Geometry check sheet. Reference: the model listing, model coordinates, mm. Face numbers are marked on the shaded views. A direction names the side the tool comes from. Give positions to 0.01 mm unless a question says otherwise; leave off trailing zeros. Write each loop counter-clockwise with the first axis right and the second up, starting at its lowest first coordinate (ties: lowest second). Pieces come first, ordered by that corner, then holes. Notation, with made-up numbers: (29, 13) - (72, 13) arc R32 ccw to (72, 48) - close; hole circle Ø9 at (88.25, 83). An arc over 180 degrees is marked (long way). One line per question, with ' | ' between items. Start each with the question number.
Q1. Section check A-A on z = 4.25. Count the separate pieces of the cut face and the enclosed holes in it, and give its area (3 significant figures).
Q2. Thickness scan on L1, parallel to X at y = 28.75, z = 6; L2, parallel to Y at x = -0.5, z = 4.5; L3, parallel to Z at x = -21.5, y = 27. Record the ranges inside material, lowest first. Write a range as [from, to].
Q3. Section check C-C on z = 9.5. Record the boundary of the cut face in (x, y), and give its area (3 significant figures).
Q4. Section check B-B on y = 0. Record the boundary of the cut face in (x, z).
Q5. Set-up check for the marked faces 1 and 2: record each of +Z, -Z, +X, -X, +Y, -Y from which the full face is reachable in a straight line by a thin tool's end or side.
Q6. Gauge pin test, flat ends, axial feed: P1, Ø3, axis at x = 10, z = 10, coming from the -Y side; P2, Ø5.5, axis at y = 25.5, z = 8, coming from the -X side; P3, Ø2, axis at y = 28, z = 9, coming from the +X side; P4, Ø19.5, axis at x = 12, y = 4, coming from the +Z side. Record the tip position at first contact, or that the pin passes through.
Q7. Section check D-D on x = -7.5. Record the boundary of the cut face in (y, z).
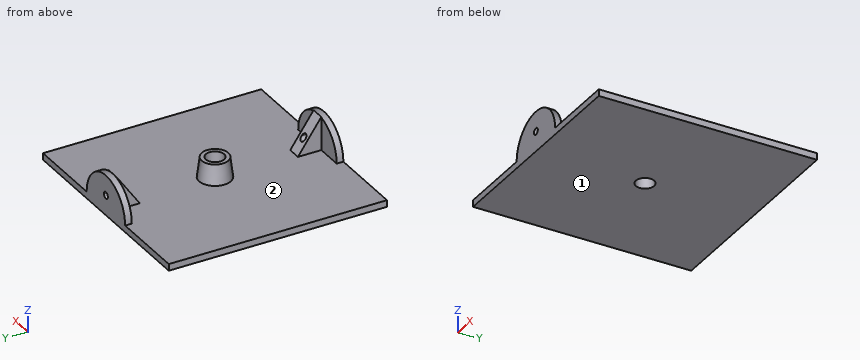
```python
from build123d import *

# Parameters (mm, degrees)
F0_W          = 65.4
F0_H          = 65.4
F1_DEPTH      = 2
F3_DEPTH      = 2
F5_DEPTH      = 2
F7_DEPTH      = 2
F7_DEPTH_BACK = 2
F9_DEPTH      = 65.401
F12_R         = 2.75
F13_DEPTH     = 8.001


with BuildPart() as f1:
    # F0 (on Top) → F1 (new body)
    with BuildSketch(Plane.XY):
        Rectangle(F0_W, F0_H)
    extrude(amount=F1_DEPTH)

    # F2 (on face) → F3 (join)
    with BuildSketch(Plane.XZ.offset(32.7)):
        with BuildLine():
            Line((-10, 2), (0, 2))
            Line((0, 2), (10, 2))
            ThreePointArc((10, 2), (0, 12), (-10, 2))
        make_face()
    extrude(amount=-F3_DEPTH)

    # F4 (on face) → F5 (join)
    with BuildSketch(Plane(origin=(0, 32.7, 0), x_dir=(-1, 0, 0), z_dir=(0, 1, 0))):
        with BuildLine():
            Line((-10, 2), (0, 2))
            Line((0, 2), (10, 2))
            ThreePointArc((10, 2), (0, 12), (-10, 2))
        make_face()
    extrude(amount=-F5_DEPTH)

    # F6 (on Right) → F7 (join, two sides)
    with BuildSketch(Plane.YZ) as f7_sk:
        Polygon((23.7, 2), (30.7, 2), (30.7, 12), align=None)
        Polygon((-23.7, 2), (-30.7, 12), (-30.7, 2), align=None)
    extrude(amount=F7_DEPTH)
    extrude(f7_sk.sketch, amount=-F7_DEPTH_BACK)

    # F8 (on face) → F9 (cut, through all)
    with BuildSketch(Plane.XZ.offset(32.7)):
        with BuildLine():
            ThreePointArc((0, 5), (0.707107, 5.292893), (1, 6))
            ThreePointArc((1, 6), (-0.707107, 6.707107), (0, 5))
        make_face()
    extrude(amount=-F9_DEPTH, mode=Mode.SUBTRACT)

    # F10 (on Front) → F11 (revolve)
    with BuildSketch(Plane.XZ):
        Polygon((0, 8), (0, 0), (5, 0), (4, 8), align=None)
    revolve(axis=Axis((0, 0, 4), (0, 0, 1)))

    # F12 (on face) → F13 (cut, through all)
    with BuildSketch(Plane.XY.offset(8)):
        Circle(F12_R)
    extrude(amount=-F13_DEPTH, mode=Mode.SUBTRACT)


solid = f1.part
```
Working result:
1) separate pieces: 3 | enclosed holes: 1 | area: 160 mm2
2) L1: x = [-2, -1], [1, 2] | L2: y = [-32.7, -25.45], [-4.41, -2.7], [2.7, 4.41], [25.45, 32.7] | L3: z = [0, 2]
3) outline: (-6.61, -32.7) - (6.61, -32.7) - (6.61, -30.7) - (2, -30.7) - (2, -28.95) - (-2, -28.95) - (-2, -30.7) - (-6.61, -30.7) - close; (-6.61, 30.7) - (-2, 30.7) - (-2, 28.95) - (2, 28.95) - (2, 30.7) - (6.61, 30.7) - (6.61, 32.7) - (-6.61, 32.7) - close | area: 66.9 mm2
4) outline: (-32.7, 0) - (-2.75, 0) - (-2.75, 8) - (-4, 8) - (-4.75, 2) - (-32.7, 2) - close; (2.75, 0) - (32.7, 0) - (32.7, 2) - (4.75, 2) - (4, 8) - (2.75, 8) - close
5) face 1: -Z, +X, -X, +Y, -Y | face 2: +Z
6) P1: passes through | P2: stops at x = -2 | P3: stops at x = 2 | P4: stops at z = 8
7) outline: (-32.7, 0) - (32.7, 0) - (32.7, 8.61) - (30.7, 8.61) - (30.7, 2) - (-30.7, 2) - (-30.7, 8.61) - (-32.7, 8.61) - close
